Verification items for the finished model (mm, model axes). Face numbers are marked on the shaded views. A direction names the side the tool comes from. Coordinates: 2 decimals unless noted, no trailing zeros. Loops run counter-clockwise (first coordinate to the right, second up) from the corner with the lowest first, then second, coordinate; pieces in that order, holes last. Notation, with made-up numbers: (25.25, 60) - (74.25, 60) arc R24 ccw to (74.25, 72) - close; hole circle Ø11 at (71.5, 88). An arc over 180 degrees is marked (long way). One line per item, written item: value. Start each with the question number.
(1) Section check B-B (x = 16.5). Record the boundary of the cut face in (y, z).
(2) Gauge pin test, flat ends, axial feed: P1, Ø3.5, axis at x = 18, z = -1.5, coming from the -Y side; P2, Ø2.5, axis at x = 2, z = -111.5, coming from the +Y side. Record the tip position at first contact, or that the pin passes through.
(3) Thickness scan on probe 1 along Z at (x, y) = (38, 39); probe 2 along X at (y, z) = (44.5, -24); probe 3 along Z at (x, y) = (24, 15.5). Record the ranges inside material, lowest first. Write a range as [from, to].
(4) Section check A-A (z = -147). Record the boundary of the cut face in (x, y).
(5) Section check D-D (y = 59). Record the boundary of the cut face in (x, z).
(6) Section check C-C (y = 28). Record the boundary of the cut face in (x, z).
(7) Set-up check for the marked faces 1 and 2: record each of +Z, -Z, +X, -X, +Y, -Y from which the full face is reachable in a straight line by a thin tool's end or side.
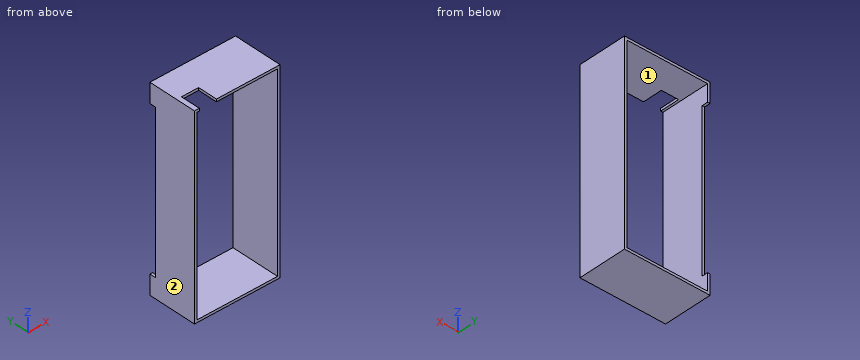
```python
from build123d import *

# Parameters (mm, degrees)
SKETCH2_W           = 111.76
SKETCH2_H           = 254
SKETCH2_W_2         = 105.156
SKETCH2_H_2         = 247.396
BOSS_EXTRUDE2_DEPTH = 63.5
SKETCH3_W           = 203.2
SKETCH3_H           = 7.62
CUT_EXTRUDE1_DEPTH  = 63.5
CUT_EXTRUDE2_REACH  = 256
SKETCH4_W           = 22.352
SKETCH4_H           = 25.4


with BuildPart() as part:
    # Sketch2 → Boss-Extrude2 (new body)
    with BuildSketch(Plane(origin=(0, 0, 0), x_dir=(1, 0, 0), z_dir=(0, 1, 0))):
        with Locations((55.88, 127)):
            Rectangle(SKETCH2_W, SKETCH2_H)
        with Locations((55.88, 127)):
            Rectangle(SKETCH2_W_2, SKETCH2_H_2, mode=Mode.SUBTRACT)
    extrude(amount=BOSS_EXTRUDE2_DEPTH)

    # Sketch3 → Cut-Extrude1 (cut)
    with BuildSketch(Plane(origin=(3.302, 0, 0), x_dir=(0, 0, -1), z_dir=(1, 0, 0))):
        with Locations((127, 59.69)):
            Rectangle(SKETCH3_W, SKETCH3_H)
    extrude(amount=-CUT_EXTRUDE1_DEPTH, mode=Mode.SUBTRACT)

    # Sketch4 → Cut-Extrude2 (cut, up to next)
    with BuildSketch(Plane.XY, mode=Mode.PRIVATE) as cut_extrude2_sk1:
        with Locations((17.526, 12.7)):
            Rectangle(SKETCH4_W, SKETCH4_H)
    cut_extrude2_tool1 = extrude(cut_extrude2_sk1.sketch, amount=-CUT_EXTRUDE2_REACH, mode=Mode.PRIVATE) & part.part
    add(cut_extrude2_tool1.solids().sort_by_distance((17.526, 12.7, 0))[0], mode=Mode.SUBTRACT)


solid = part.part
```
Responses:
1. outline: (0, -254) - (63.5, -254) - (63.5, -250.7) - (0, -250.7) - close; (25.4, -3.3) - (63.5, -3.3) - (63.5, 0) - (25.4, 0) - close
2. P1: stops at y = 25.4
2. P2: stops at y = 55.88
3. probe 1: z = [-254, -250.7], [-3.3, 0]
3. probe 2: x = [0, 3.3], [108.46, 111.76]
3. probe 3: z = [-254, -250.7]
4. outline: (0, 0) - (3.3, 0) - (3.3, 55.88) - (0, 55.88) - close; (108.46, 0) - (111.76, 0) - (111.76, 63.5) - (108.46, 63.5) - close
5. outline: (0, -254) - (111.76, -254) - (111.76, 0) - (0, 0) - (0, -25.4) - (3.3, -25.4) - (3.3, -3.3) - (108.46, -3.3) - (108.46, -250.7) - (3.3, -250.7) - (3.3, -228.6) - (0, -228.6) - close
6. outline: (0, -254) - (111.76, -254) - (111.76, 0) - (0, 0) - close; hole (3.3, -250.7) - (108.46, -250.7) - (108.46, -3.3) - (3.3, -3.3) - close
7. face 1: +Y, -Y
7. face 2: +Z, -Z, -X, +Y, -Y
